Work out the finished part from the listing and answer in its coordinate system (mm). A direction names the side the tool comes from. Coordinates: 2 decimals unless noted, no trailing zeros. Loops run counter-clockwise (first coordinate to the right, second up) from the corner with the lowest first, then second, coordinate; pieces in that order, holes last.
```python
from build123d import *

# Parameters (mm, degrees)
CROQUIS1_R                   = 6
SALIENTE_EXTRUIR1_DEPTH      = 250
SALIENTE_EXTRUIR2_DEPTH      = 10
SALIENTE_EXTRUIR2_DEPTH_BACK = 2
CROQUIS2_R                   = 7.5
SALIENTE_EXTRUIR3_DEPTH      = 10
SALIENTE_EXTRUIR3_DEPTH_BACK = 2
CROQUIS3_R                   = 7.5
SALIENTE_EXTRUIR4_DEPTH      = 2
SALIENTE_EXTRUIR5_DEPTH      = 2


with BuildPart() as part:
    # Croquis1 → Saliente-Extruir1 (new body)
    with BuildSketch(Plane.XY):
        Circle(CROQUIS1_R)
    extrude(amount=SALIENTE_EXTRUIR1_DEPTH)

    # Croquis2 → Saliente-Extruir2 (add, two sides: drawn at the far end of the back side and taken through both)
    with BuildSketch(Plane.XY.offset(250).offset(-SALIENTE_EXTRUIR2_DEPTH_BACK)):
        Circle(CROQUIS2_R)
    extrude(amount=SALIENTE_EXTRUIR2_DEPTH + SALIENTE_EXTRUIR2_DEPTH_BACK)

    # Croquis3 → Saliente-Extruir3 (add, two sides: drawn at the far end of the back side and taken through both)
    with BuildSketch(Plane(origin=(0, 0, 0), x_dir=(-1, 0, 0), z_dir=(0, 0, -1)).offset(-SALIENTE_EXTRUIR3_DEPTH_BACK)):
        with Locations(Location((0, 0, 0), (0, 0, 180))):
            Circle(CROQUIS3_R)
    extrude(amount=SALIENTE_EXTRUIR3_DEPTH + SALIENTE_EXTRUIR3_DEPTH_BACK)

    # Croquis4 → Saliente-Extruir4 (add)
    with BuildSketch(Plane.XY.offset(260)):
        Polygon((3.464101615, 0), (1.732050808, 3), (-1.732050808, 3), (-3.464101615, 0), (-1.732050808, -3), (1.732050808, -3), align=None)
    extrude(amount=SALIENTE_EXTRUIR4_DEPTH)

    # Croquis5 → Saliente-Extruir5 (add)
    with BuildSketch(Plane(origin=(0, 0, -10), x_dir=(-1, 0, 0), z_dir=(0, 0, -1))):
        Polygon((1.963176251, 2.854109144), (-1.490142898, 3.127215078), (-3.45331915, 0.273105934), (-1.963176251, -2.854109144), (1.490142898, -3.127215078), (3.45331915, -0.273105934), align=None)
    extrude(amount=SALIENTE_EXTRUIR5_DEPTH)


solid = part.part
```
1. A cutting plane is placed at A-A, the plane z = 184.5. Give the vertices of the cut face in (x, y).
2. Each of these flat-tipped pins is pushed along its axis until it touches: P1, Ø0.6, axis at x = 0, z = 261.5, coming from the +Y side; P2, Ø6, axis at x = 0.5, z = 106.5, coming from the +Y side; P3, Ø5, axis at x = 6, z = 121.5, coming from the -Y side. Where does it stop, or does it pass through?
3. For faces 1 (the flat face through (0, 0, -12)), 2 (the flat face through (-0.1, -3.2, 260)), 3 (the flat face through (-0.1, 3.2, -10)), 4 (the cylindrical face through (-7.493, 0.33, 253.916)), 5 (the flat face through (2, -6, 2)), determine the directions among +Z, -Z, +X, -X, +Y, -Y from which every point of the face is accessible in a straight line to the end or side of a thin tool.
4. Straight lines are drawn through the part: probe 1 along Z at (x, y) = (-2.25, -5.75); probe 2 along Z at (x, y) = (-0.25, -3.25); probe 3 along Y at (x, z) = (5.25, 206). For each, find the intervals that lie inside material, in ascending order.
5. Determine the mould class of faces 6 (the cylindrical face through (-6, 0, 123)), 7 (the cylindrical face through (4.032, -6.324, -3.916)), 8 (the flat face through (0, 0, 262)), 9 (the flat face through (2, 6, 248)) for opening direction Z: released by +Z, released by -Z, zero draft, split by the parting line, or undercut.
Answers below:
1. outline: circle Ø12 at (0, 0)
2. P1: stops at y = 3
2. P2: stops at y = 6
2. P3: stops at y = -4.87
3. face 1: -Z, +X, -X, +Y, -Y
3. face 2: +Z
3. face 3: -Z
3. face 4: +Z, -Z
3. face 5: none
4. probe 1: z = -10 to 2, 248 to 260
4. probe 2: z = -10 to 260
4. probe 3: y = -2.9 to 2.9
5. face 6: undercut
5. face 7: zero draft
5. face 8: released by +Z
5. face 9: undercut
